Can you work these out from the model? Positions are in its coordinate system, mm. A direction names the side the tool comes from. Give positions to 0.01 mm unless a question says otherwise; leave off trailing zeros. Loops run counter-clockwise (first coordinate to the right, second up) from the corner with the lowest first, then second, coordinate; pieces in that order, holes last.
from build123d import *

# Parameters (mm, degrees)
F0_R         = 3.95
F1_DEPTH     = 120
F3_DEPTH     = 120.001
F4_R         = 1
F5_DEPTH     = 25
F6_W         = 2
F6_H         = 40
F7_DEPTH     = 4
F8_T1_DEPTH  = 45
F8_T6_DEPTH  = 22.5
F8_S7_R      = 1
F8_T8_DEPTH  = 13
F8_T12_DEPTH = 22.5
F8_S13_R     = 1
F8_T14_DEPTH = 13
F8_T18_DEPTH = 22.5
F8_S19_R     = 1
F8_T20_DEPTH = 13
F8_T24_DEPTH = 22.5
F8_S25_R     = 1
F8_T26_DEPTH = 13


# Not quite as in the source:
# - a fillet or chamfer that OpenCascade refuses, or shapes differently, is made with other operations: its cross-section is extruded or revolved along the edge and cut away or added


with BuildPart() as f1:
    # F0 (on Top) → F1 (new body)
    with BuildSketch(Plane.XY):
        Circle(F0_R)
    extrude(amount=F1_DEPTH)

    # F2 (on face) → F3 (cut, through all)
    with BuildSketch(Plane.XY.offset(120)):
        with BuildLine():
            Line((-2.8354893758, -2.75), (-2.8354893758, 2.75))
            ThreePointArc((-2.8354893758, 2.75), (-3.95, 0), (-2.8354893758, -2.75))
        make_face()
        with BuildLine():
            ThreePointArc((3.95, 0), (3.6607842762, 1.4836301705), (2.8354893758, 2.75))
            Line((2.8354893758, 2.75), (2.8354893758, -2.75))
            ThreePointArc((2.8354893758, -2.75), (3.6607842762, -1.4836301705), (3.95, 0))
        make_face()
    extrude(amount=-F3_DEPTH, mode=Mode.SUBTRACT)

    # F4 (on face) → F5 (join)
    with BuildSketch(Plane.XY.offset(120)):
        Circle(F4_R)
    extrude(amount=F5_DEPTH)

    # F6 (on face) → F7 (join)
    with BuildSketch(Plane.XY.offset(145)):
        Rectangle(F6_W, F6_H)
    extrude(amount=F7_DEPTH)

    # F8: fillet of radius 1 on 6 edges, made by hand

    # F8_s2 → F8_t1 (cut)
    with BuildSketch(Plane.XZ.offset(-22.5)):
        with BuildLine():
            ThreePointArc((1, 148), (0.7071067812, 148.7071067812), (0, 149))
            Line((0, 149), (1, 149))
            Line((1, 149), (1, 148))
        make_face()
        with BuildLine():
            ThreePointArc((-1, 148), (-0.7071067812, 148.7071067812), (0, 149))
            Line((0, 149), (-1, 149))
            Line((-1, 149), (-1, 148))
        make_face()
    extrude(amount=F8_T1_DEPTH, mode=Mode.SUBTRACT)


with BuildPart() as f8_tool4:
    # F8_s5 → F8_t6 (new body)
    with BuildSketch(Plane.XZ.offset(22.5)):
        with BuildLine():
            ThreePointArc((0, 145), (0.7071067812, 145.2928932188), (1, 146))
            Line((1, 146), (1, 145))
            Line((1, 145), (0, 145))
        make_face()
    extrude(amount=-F8_T6_DEPTH)

    # F8_s7 → F8_t8 (cut, symmetric)
    with BuildSketch(Plane.XY.offset(145.5)):
        Circle(F8_S7_R)
    extrude(amount=F8_T8_DEPTH, both=True, mode=Mode.SUBTRACT)


with BuildPart() as f1_1:
    add(f1.part)

    # F8_t3: cut F8_tool4
    add(f8_tool4.part, mode=Mode.SUBTRACT)


with BuildPart() as f8_tool10:
    # F8_s11 → F8_t12 (new body)
    with BuildSketch(Plane.XZ):
        with BuildLine():
            ThreePointArc((0, 145), (-0.7071067812, 145.2928932188), (-1, 146))
            Line((-1, 146), (-1, 145))
            Line((-1, 145), (0, 145))
        make_face()
    extrude(amount=F8_T12_DEPTH)

    # F8_s13 → F8_t14 (cut, symmetric)
    with BuildSketch(Plane.XY.offset(145.5)):
        Circle(F8_S13_R)
    extrude(amount=F8_T14_DEPTH, both=True, mode=Mode.SUBTRACT)


with BuildPart() as f1_2:
    add(f1_1.part)

    # F8_t9: cut F8_tool10
    add(f8_tool10.part, mode=Mode.SUBTRACT)


with BuildPart() as f8_tool16:
    # F8_s17 → F8_t18 (new body)
    with BuildSketch(Plane.XZ.offset(-22.5)):
        with BuildLine():
            ThreePointArc((0, 145), (-0.7071067812, 145.2928932188), (-1, 146))
            Line((-1, 146), (-1, 145))
            Line((-1, 145), (0, 145))
        make_face()
    extrude(amount=F8_T18_DEPTH)

    # F8_s19 → F8_t20 (cut, symmetric)
    with BuildSketch(Plane.XY.offset(145.5)):
        Circle(F8_S19_R)
    extrude(amount=F8_T20_DEPTH, both=True, mode=Mode.SUBTRACT)


with BuildPart() as f1_3:
    add(f1_2.part)

    # F8_t15: cut F8_tool16
    add(f8_tool16.part, mode=Mode.SUBTRACT)


with BuildPart() as f8_tool22:
    # F8_s23 → F8_t24 (new body)
    with BuildSketch(Plane.XZ):
        with BuildLine():
            ThreePointArc((0, 145), (0.7071067812, 145.2928932188), (1, 146))
            Line((1, 146), (1, 145))
            Line((1, 145), (0, 145))
        make_face()
    extrude(amount=-F8_T24_DEPTH)

    # F8_s25 → F8_t26 (cut, symmetric)
    with BuildSketch(Plane.XY.offset(145.5)):
        Circle(F8_S25_R)
    extrude(amount=F8_T26_DEPTH, both=True, mode=Mode.SUBTRACT)


with BuildPart() as f1_4:
    add(f1_3.part)

    # F8_t21: cut F8_tool22
    add(f8_tool22.part, mode=Mode.SUBTRACT)


solid = f1_4.part
(1) Which directions (+Z, -Z, +X, -X, +Y, -Y) give clear straight access to the entire face, cutting with the end or side of a thin tool? Please do faces 4 (the cylindrical face through (-0.04, -3.95, 59.16)), 5 (the cylindrical face through (0.04, 3.95, 59.16)), 6 (the flat face through (-2.835, 0, 61)).
Returned:
face 4: -Z, -Y
face 5: -Z, +Y
face 6: +Z, -Z, -X, +Y, -Y
(2) Will these pins go through, and if not, where does the flat tip stop? P1, Ø1.5, axis at y = -6, z = 36.5, coming from the +X side; P2, Ø3, axis at x = -2, y = 10.5, coming from the -Z side; P3, Ø0.6, axis at y = 5, z = 146.5, coming from the +X side; P4, Ø2, axis at x = -1, z = 96.5, coming from the -Y side.
Returned:
P1: passes through
P2: stops at z = 145.13
P3: stops at x = 1
P4: stops at y = -3.95
(3) Suppose I cut it at C-C on z = 49.5. List the corners of the cut face in (x, y) for me, plus the area to 3 significant figures.
Returned:
outline: (-2.84, -2.75) arc R3.95 ccw to (2.84, -2.75) - (2.84, 2.75) arc R3.95 ccw to (-2.84, 2.75) - close
area: 40.6 mm2
(4) Please list where these lines run through material, in increasing order: probe 1 along Y at (x, z) = (-0.25, 13); probe 2 along Y at (x, z) = (-0.1, 134); probe 3 along Z at (x, y) = (0.2, -0.5).
Returned:
probe 1: y = -3.94 to 3.94
probe 2: y = -0.99 to 0.99
probe 3: z = 0 to 148.98
(5) Suppose I cut it at A-A on y = -10. List the corners of the cut face in (x, z) for me.
Returned:
outline: (-1, 146) arc R1 ccw to (1, 146) - (1, 148) arc R1 ccw to (-1, 148) - close
(6) Thinking about a two-plate mould opening in Z: for faces 1 (the flat face through (0, 0, 0)), 2 (the flat face through (1, -1, 120)), 3 (the flat face through (2.835, 0, 61)), which applies, pulls with the +Z half, pulls with the -Z half, needs draft (parallel to the pull), parting line crosses it, or undercut?
Returned:
face 1: pulls with the -Z half
face 2: undercut
face 3: needs draft
(7) Suppose I cut it at B-B on z = 140. List the corners of the cut face in (x, y) for me, plus the area to 3 significant figures.
Returned:
outline: circle Ø2 at (0, 0)
area: 3.14 mm2
